Design review of the part built by this model. Coordinates are the model's own, in mm. Face numbers are marked on the shaded views. A direction names the side the tool comes from. Coordinates: 2 decimals unless noted, no trailing zeros. Order: outer loops, then holes, each group sorted by start corner. A loop starts at its lowest first (then second) coordinate and runs counter-clockwise, first axis right, second up. Notation, with made-up numbers: M -14.75,3.25 L 10.25,3.25 A20 ccw 10.25,17.25 Z; hole C 22,-11 d2. An arc over 180 degrees is marked long. Answer in a Markdown table with one row per item.
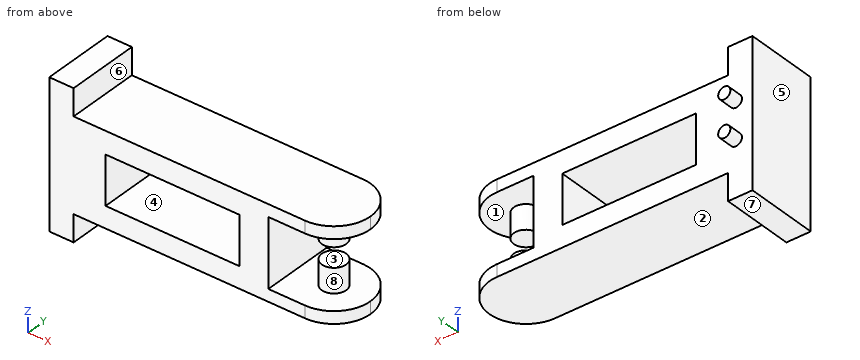
from build123d import *

# Parameters (mm, degrees)
BOSS_EXTRUDE1_DEPTH      = 15
BOSS_EXTRUDE1_DEPTH_BACK = 15
CUT_EXTRUDE1_DEPTH       = 38
SKETCH6_W                = 55
SKETCH6_H                = 20
CUT_EXTRUDE2_DEPTH       = 38
SKETCH8_R                = 5
BOSS_EXTRUDE2_DEPTH      = 10
SKETCH9_R                = 2.5
BOSS_EXTRUDE3_DEPTH      = 6


with BuildPart() as part:
    # Sketch1 → Boss-Extrude1 (new body, two sides)
    with BuildSketch(Plane(origin=(0, 0, 0), x_dir=(1, 0, 0), z_dir=(0, 1, 0))) as boss_extrude1_sk:
        Polygon((-13.124974518, 30), (-13.124974518, 19), (96.875025482, 19), (96.875025482, 14), (66.875025482, 14), (66.875025482, -14), (96.875025482, -14), (96.875025482, -19), (-13.124974518, -19), (-13.124974518, -30), (-23.124974518, -30), (-23.124974518, 30), align=None)
    extrude(amount=BOSS_EXTRUDE1_DEPTH)
    extrude(boss_extrude1_sk.sketch, amount=-BOSS_EXTRUDE1_DEPTH_BACK)

    # Sketch4 → Cut-Extrude1 (cut)
    with BuildSketch(Plane.XY.offset(19)):
        with BuildLine():
            Line((96.875025482, 15), (81.875025482, 15))
            ThreePointArc((81.875025482, 15), (92.4816272, 10.606601718), (96.875025482, 0))
            Line((96.875025482, 0), (96.875025482, 15))
        make_face()
        with BuildLine():
            Line((96.875025482, -15), (96.875025482, 0))
            ThreePointArc((96.875025482, 0), (92.4816272, -10.606601718), (81.875025482, -15))
            Line((81.875025482, -15), (96.875025482, -15))
        make_face()
    extrude(amount=-CUT_EXTRUDE1_DEPTH, mode=Mode.SUBTRACT)

    # Sketch6 → Cut-Extrude2 (cut)
    with BuildSketch(Plane(origin=(0, 15, 0), x_dir=(1, 0, 0), z_dir=(0, 1, 0))):
        with Locations((27.5, 0.205975337)):
            Rectangle(SKETCH6_W, SKETCH6_H)
    extrude(amount=-CUT_EXTRUDE2_DEPTH, mode=Mode.SUBTRACT)

    # Sketch8 → Boss-Extrude2 (add)
    with BuildSketch(Plane(origin=(0, 0, 14), x_dir=(-1, 0, 0), z_dir=(0, 0, -1))):
        with Locations((-81.875025482, 0)):
            Circle(SKETCH8_R)
    boss_extrude2 = extrude(amount=BOSS_EXTRUDE2_DEPTH)

    # Mirror1: Boss-Extrude2 across plane
    add(boss_extrude2.mirror(Plane.XY))

    # Sketch9 → Boss-Extrude3 (add)
    with BuildSketch(Plane(origin=(0, 15, 0), x_dir=(1, 0, 0), z_dir=(0, 1, 0))):
        with Locations((-16.320792203, 7.5)):
            Circle(SKETCH9_R)
        with Locations((-16.320792203, -7.5)):
            Circle(SKETCH9_R)
    extrude(amount=BOSS_EXTRUDE3_DEPTH)


solid = part.part
(1) Add section C-C, the plane z = -1. Give the boundary of the cut face in (x, y).
Return value:
| item | result |
|---|---|
| outline | M -23.12,-15 L 0,-15 L 0,15 L -23.12,15 Z; M 55,-15 L 66.88,-15 L 66.88,15 L 55,15 Z |
(2) Add section D-D, the plane y = 7. Give the boundary of the cut face in (x, z).
Return value:
| item | result |
|---|---|
| outline | M -23.12,-30 L -13.12,-30 L -13.12,-19 L 95.14,-19 L 95.14,-14 L 66.88,-14 L 66.88,14 L 95.14,14 L 95.14,19 L -13.12,19 L -13.12,30 L -23.12,30 Z; hole M 0,-10.21 L 55,-10.21 L 55,9.79 L 0,9.79 Z |
(3) Add section A-A, the plane x = 52.5. Give the boundary of the cut face in (y, z), and give its area (3 significant figures).
Return value:
| item | result |
|---|---|
| outline | M -15,-19 L 15,-19 L 15,-10.21 L -15,-10.21 Z; M -15,9.79 L 15,9.79 L 15,19 L -15,19 Z |
| area | 540 mm2 |
(4) Draft analysis for pull direction Z (two halves, no side actions). For the marked faces 6, 7 and 8, state which applies: pulls with the +Z half, pulls with the -Z half, needs draft (parallel to the pull), parting line crosses it, or undercut.
Return value:
| item | result |
|---|---|
| face 6 | needs draft |
| face 7 | pulls with the -Z half |
| face 8 | undercut |
(5) For line 1 along Z through (x, y) = (41, 10); line 2 along X through (y, z) = (-4, 3); line 3 along Z through (x, y) = (74.5, 12), list the stretches that pass through material, from the lowest coordinate up. Write a range as from..to.
Return value:
| item | result |
|---|---|
| line 1 | z = -19..-10.21, 9.79..19 |
| line 2 | x = -23.12..0, 55..66.88 |
| line 3 | z = -19..-14, 14..19 |
(6) For the marked faces 1, 2, 3, 4 and 5, list the 3-axis set-ups (+Z, -Z, +X, -X, +Y, -Y) from which the entire face can be reached by the end or side of a thin tool; tool diameter is ignored.
Return value:
| item | result |
|---|---|
| face 1 | none |
| face 2 | -Z, +X, +Y, -Y |
| face 3 | +X, +Y, -Y |
| face 4 | +Y, -Y |
| face 5 | +Z, -Z, -X, +Y, -Y |
(7) Insertion check: pin 1 Ø1 at (y, z) = (-1.5, 20.5) entering from +X (3 decimals); pin 2 Ø5 at (x, y) = (81.5, -1) entering from +Z; pin 3 Ø5 at (x, z) = (66.5, -1.5) entering from +Y. Each pin has a flat end and moves straight along its axis. Give the tip position at first contact, or say it passes through.
Return value:
| item | result |
|---|---|
| pin 1 | stops at x = -13.125 |
| pin 2 | stops at z = 19 |
| pin 3 | stops at y = 15 |
(8) Add section B-B, the plane z = 7.5. Give the boundary of the cut face in (x, y).
Return value:
| item | result |
|---|---|
| outline | M -23.12,-15 L 0,-15 L 0,15 L -13.82,15 L -13.82,21 L -18.82,21 L -18.82,15 L -23.12,15 Z; M 55,-15 L 66.88,-15 L 66.88,15 L 55,15 Z; C 81.88,0 d10 |
